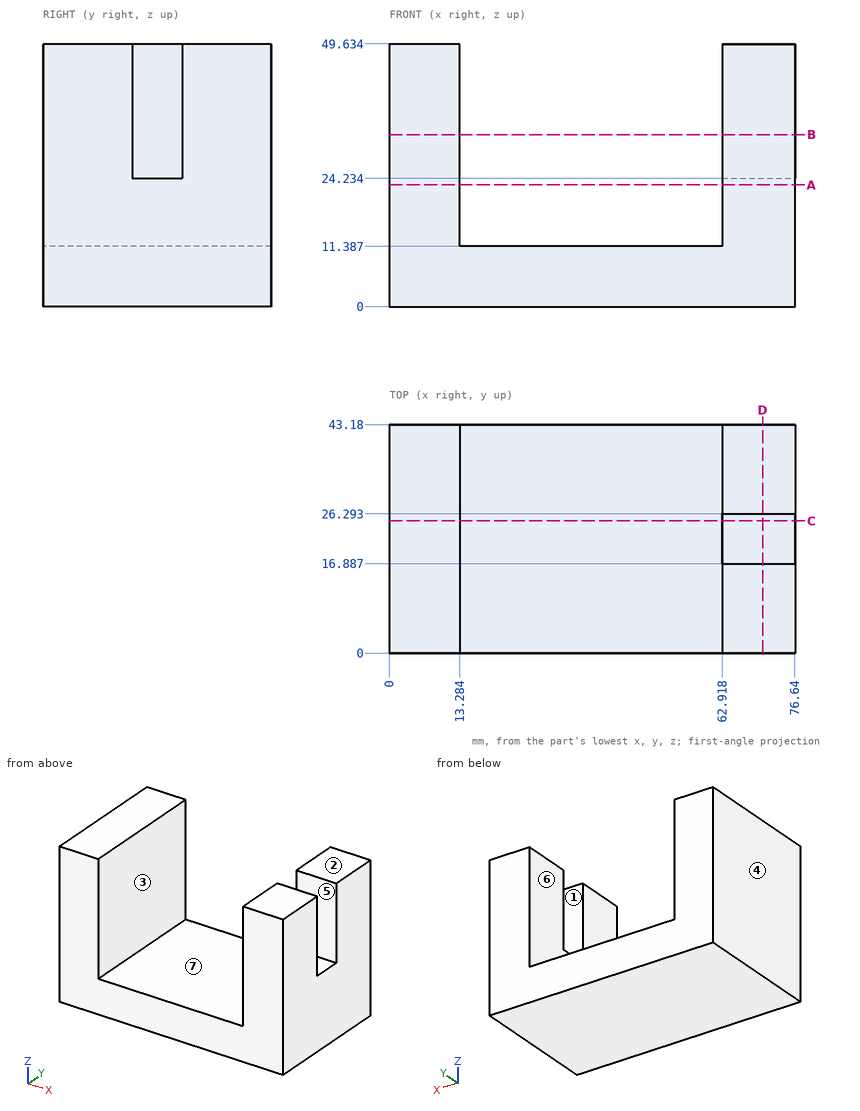
Design review of the part shown in the three views and the two pictorial views. Dimensions are in mm from the part's minimum x, y and z. A direction names the side the tool comes from. Give positions to 0.01 mm unless a question says otherwise; leave off trailing zeros. Loops run counter-clockwise (first coordinate to the right, second up) from the corner with the lowest first, then second, coordinate; pieces in that order, holes last. Notation, with made-up numbers: M -17.75,-7 L 9.25,-7 A32 ccw 9.25,31 Z; hole C 32,82.5 d9. An arc over 180 degrees is marked long. Answer as a JSON object with one key per item and string values.
Item 1: We need section D-D (x = 70.5). State the section outline as (y, z) points, and give its area (3 significant figures).
Output values:
{"outline": "M 0,0 L 43.18,0 L 43.18,49.63 L 26.29,49.63 L 26.29,24.23 L 16.89,24.23 L 16.89,49.63 L 0,49.63 Z", "area": "1,900 mm2"}
Item 2: Mouldability with a two-part tool opening along X and no side actions: class the marked faces 4, 5, 6 and 7 as pulls with the +X half, pulls with the -X half, needs draft (parallel to the pull), parting line crosses it, or undercut.
Output values:
{"face 4": "pulls with the -X half", "face 5": "needs draft", "face 6": "undercut", "face 7": "undercut"}
Item 3: Machinability: for the marked faces 1, 2 and 3, which of the approach directions +Z, -Z, +X, -X, +Y, -Y give a long, thin tool a straight path to every point of the face, cutting with its end or side? Answer none if there is none.
Output values:
{"face 1": "+Z, +X", "face 2": "+Z, +X, -X, +Y, -Y", "face 3": "+Z, +Y, -Y"}
Item 4: For P1, Ø21.5, axis at x = 37.5, y = 20.5, coming from the +Z side; P2, Ø3, axis at x = 68.5, y = 22, coming from the +Z side, all flat-tipped, find the tip position at first contact; note any pin that passes through.
Output values:
{"P1": "stops at z = 11.39", "P2": "stops at z = 24.23"}
Item 5: We need section A-A (z = 23). State the section outline as (x, y) points (1 decimal).
Output values:
{"outline": "M 0,0 L 13.3,0 L 13.3,43.2 L 0,43.2 Z; M 62.9,0 L 76.6,0 L 76.6,43.2 L 62.9,43.2 Z"}
Item 6: We need section B-B (z = 32.5). State the section outline as (x, y) points (1 decimal), and give its area (3 significant figures).
Output values:
{"outline": "M 0,0 L 13.3,0 L 13.3,43.2 L 0,43.2 Z; M 62.9,0 L 76.6,0 L 76.6,16.9 L 62.9,16.9 Z; M 62.9,26.3 L 76.6,26.3 L 76.6,43.2 L 62.9,43.2 Z", "area": "1,040 mm2"}
Item 7: Wall thickness on line 1 along X through (y, z) = (36, 41.5) (1 decimal); line 2 along Y through (x, z) = (71, 27.5); line 3 along Z through (x, y) = (22.5, 33): over which ranges is each line inside the solid? List them lowest first.
Output values:
{"line 1": "x = 0 to 13.3, 62.9 to 76.6", "line 2": "y = 0 to 16.89, 26.29 to 43.18", "line 3": "z = 0 to 11.39"}
Item 8: We need section C-C (y = 25). State the section outline as (x, z) points (1 decimal).
Output values:
{"outline": "M 0,0 L 76.6,0 L 76.6,24.2 L 62.9,24.2 L 62.9,11.4 L 13.3,11.4 L 13.3,49.6 L 0,49.6 Z"}
